```python
from build123d import *

# Parameters (mm, degrees)
SKETCH1_R           = 2.5
BOSS_EXTRUDE1_DEPTH = 50


with BuildPart() as part:
    # Sketch1 → Boss-Extrude1 (new body)
    with BuildSketch(Plane(origin=(0, 0, 0), x_dir=(0, 0, -1), z_dir=(1, 0, 0))):
        with BuildLine():
            Line((-0.450054938, 23), (-1, 22.331430068))
            Line((-1, 22.331430068), (-1, 21.476731595))
            ThreePointArc((-1, 21.476731595), (-8.227693796, 19.863409949), (-14.479235767, 15.89344933))
            Line((-14.479235767, 15.89344933), (-14.695203551, 15.693979501))
            Line((-14.695203551, 15.693979501), (-14.925214831, 16.339428393))
            Line((-14.925214831, 16.339428393), (-15.556349186, 16.970562748))
            Line((-15.556349186, 16.970562748), (-16.581692866, 15.945219069))
            Line((-16.581692866, 15.945219069), (-16.497812416, 15.083598853))
            Line((-16.497812416, 15.083598853), (-15.89344933, 14.479235767))
            ThreePointArc((-15.89344933, 14.479235767), (-19.863409949, 8.227693796), (-21.476731595, 1))
            Line((-21.476731595, 1), (-21.488397411, 0.706241247))
            Line((-21.488397411, 0.706241247), (-22.107441235, 1))
            Line((-22.107441235, 1), (-23, 1))
            Line((-23, 1), (-23, -0.450054938))
            Line((-23, -0.450054938), (-22.331430068, -1))
            Line((-22.331430068, -1), (-21.476731595, -1))
            ThreePointArc((-21.476731595, -1), (-19.863409949, -8.227693796), (-15.89344933, -14.479235767))
            Line((-15.89344933, -14.479235767), (-15.693979501, -14.695203551))
            Line((-15.693979501, -14.695203551), (-16.339428393, -14.925214831))
            Line((-16.339428393, -14.925214831), (-16.970562748, -15.556349186))
            Line((-16.970562748, -15.556349186), (-15.945219069, -16.581692866))
            Line((-15.945219069, -16.581692866), (-15.083598853, -16.497812416))
            Line((-15.083598853, -16.497812416), (-14.479235767, -15.89344933))
            ThreePointArc((-14.479235767, -15.89344933), (-8.227693796, -19.863409949), (-1, -21.476731595))
            Line((-1, -21.476731595), (-0.706241247, -21.488397411))
            Line((-0.706241247, -21.488397411), (-1, -22.107441235))
            Line((-1, -22.107441235), (-1, -23))
            Line((-1, -23), (0.450054938, -23))
            Line((0.450054938, -23), (1, -22.331430068))
            Line((1, -22.331430068), (1, -21.476731595))
            ThreePointArc((1, -21.476731595), (8.227693796, -19.863409949), (14.479235767, -15.89344933))
            Line((14.479235767, -15.89344933), (14.695203551, -15.693979501))
            Line((14.695203551, -15.693979501), (14.925214831, -16.339428393))
            Line((14.925214831, -16.339428393), (15.556349186, -16.970562748))
            Line((15.556349186, -16.970562748), (16.581692866, -15.945219069))
            Line((16.581692866, -15.945219069), (16.497812416, -15.083598853))
            Line((16.497812416, -15.083598853), (15.89344933, -14.479235767))
            ThreePointArc((15.89344933, -14.479235767), (19.863409949, -8.227693796), (21.476731595, -1))
            Line((21.476731595, -1), (21.488397411, -0.706241247))
            Line((21.488397411, -0.706241247), (22.107441235, -1))
            Line((22.107441235, -1), (23, -1))
            Line((23, -1), (23, 0.450054938))
            Line((23, 0.450054938), (22.331430068, 1))
            Line((22.331430068, 1), (21.476731595, 1))
            ThreePointArc((21.476731595, 1), (19.863409949, 8.227693796), (15.89344933, 14.479235767))
            Line((15.89344933, 14.479235767), (15.693979501, 14.695203551))
            Line((15.693979501, 14.695203551), (16.339428393, 14.925214831))
            Line((16.339428393, 14.925214831), (16.970562748, 15.556349186))
            Line((16.970562748, 15.556349186), (15.945219069, 16.581692866))
            Line((15.945219069, 16.581692866), (15.083598853, 16.497812416))
            Line((15.083598853, 16.497812416), (14.479235767, 15.89344933))
            ThreePointArc((14.479235767, 15.89344933), (8.227693796, 19.863409949), (1, 21.476731595))
            Line((1, 21.476731595), (0.706241247, 21.488397411))
            Line((0.706241247, 21.488397411), (1, 22.107441235))
            Line((1, 22.107441235), (1, 23))
            Line((1, 23), (-0.450054938, 23))
        make_face()
        Circle(SKETCH1_R, mode=Mode.SUBTRACT)
    extrude(amount=BOSS_EXTRUDE1_DEPTH)


solid = part.part
```
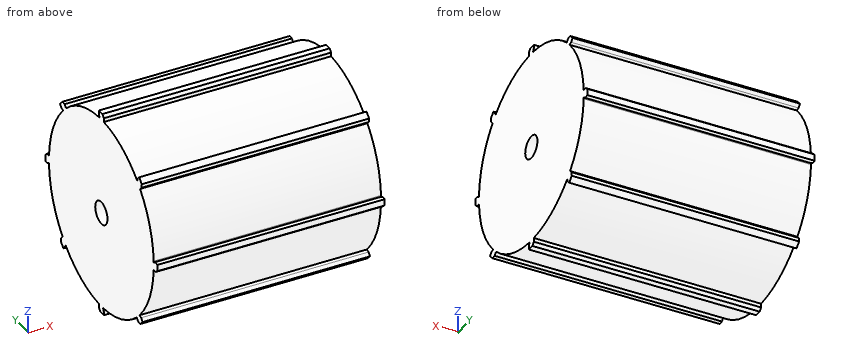
Can you work these out from the model? Positions are in its coordinate system, mm. Give positions to 0.01 mm unless a question says otherwise; leave off trailing zeros. Write each loop counter-clockwise with the first axis right and the second up, starting at its lowest first coordinate (ties: lowest second). Pieces come first, ordered by that corner, then holes. Notation, with made-up numbers: (76.5, -20) -> (110.5, -20) arc R23 ccw to (110.5, -8) -> close; hole circle Ø9 at (-17, 23). An arc over 180 degrees is marked (long way). Write item = value, one per line.
(1) Suppose I cut it at B-B on y = -3.5. Write out the boundary of the cut face in (x, z), then the cut area to 3 significant figures.
Worked out:
outline = (0, -21.21) -> (50, -21.21) -> (50, 21.21) -> (0, 21.21) -> close
area = 2,120 mm^2
(2) I need wall thicknesses on probe 1 along Y at (x, z) = (39.5, 0); probe 2 along Z at (x, y) = (45, -16); probe 3 along Z at (x, y) = (16.5, 0.5). Which ranges of each line are inside material? Lowest first, please. Write a range as from..to.
Worked out:
probe_1 = -23..-2.5, 2.5..23
probe_2 = -16.53..-14.8, -14.36..14.36, 14.59..16.53
probe_3 = -22.94..-2.45, 2.45..23
(3) Suppose I cut it at A-A on y = -12. Write out the boundary of the cut face in (x, z).
Worked out:
outline = (0, -17.84) -> (50, -17.84) -> (50, 17.84) -> (0, 17.84) -> close
(4) I'm going to push flat-ended pins straight in: P1, Ø0.9, axis at x = 23.5, z = -22, coming from the +Y side; P2, Ø0.7, axis at x = 18.5, z = 22, coming from the -Y side; P3, Ø0.9, axis at x = 28, y = -22, coming from the -Z side. Where does each tip first touch, or does it pass through?
Worked out:
P1 = 1
P2 = -1
P3 = -1
